Could you check a few things on this model? Use its own coordinates, in mm. Give positions to 0.01 mm unless a question says otherwise; leave off trailing zeros. Order: outer loops, then holes, each group sorted by start corner. A loop starts at its lowest first (then second) coordinate and runs counter-clockwise, first axis right, second up. Notation, with made-up numbers: M 9,11 L 51,11 A21 cw 51,44 Z; hole C 15,80 d11. An arc over 180 degrees is marked long. Answer in a Markdown table with one row per item. Add a question column.
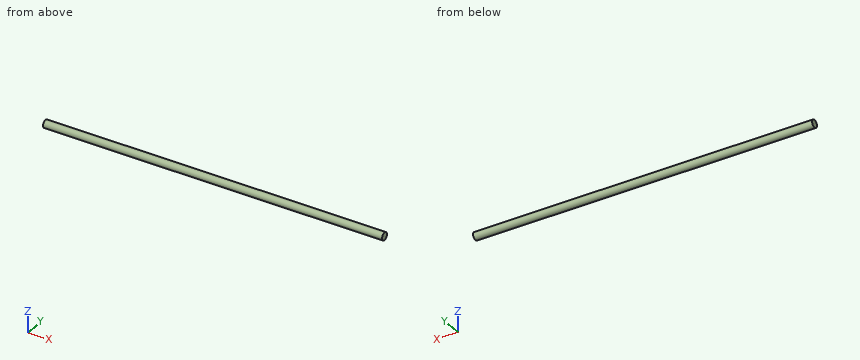
```python
from build123d import *

# Parameters (mm, degrees)
F0_R          = 59.6501704978
F1_DEPTH      = 304.8
F1_DEPTH_BACK = 304.8
F2_R          = 59.6501704978
F2_R_2        = 21.0714216583
F3_DEPTH      = 609.601
F4_R          = 21.0714216583
F4_R_2        = 8.5899800626
F5_DEPTH      = 609.601
F6_DEPTH      = 152.4
F7_DEPTH      = 152.4
F8_DEPTH      = 76.2
F9_DEPTH      = 76.2


with BuildPart() as f1:
    # F0 (on Right) → F1 (new body, two sides)
    with BuildSketch(Plane.YZ) as f1_sk:
        Circle(F0_R)
    extrude(amount=F1_DEPTH)
    extrude(f1_sk.sketch, amount=-F1_DEPTH_BACK)

    # F2 (on face) → F3 (cut, through all)
    with BuildSketch(Plane.YZ.offset(304.8)):
        Circle(F2_R)
        Circle(F2_R_2, mode=Mode.SUBTRACT)
    extrude(amount=-F3_DEPTH, mode=Mode.SUBTRACT)

    # F4 (on face) → F5 (cut, through all)
    with BuildSketch(Plane.YZ.offset(304.8)):
        Circle(F4_R)
        Circle(F4_R_2, mode=Mode.SUBTRACT)
    extrude(amount=-F5_DEPTH, mode=Mode.SUBTRACT)

    # F6 (add): a face of the model
    f6_faces = [f1.faces().sort_by_distance(p)[0] for p in [
        (304.8, 0, 0),
    ]]
    extrude(f6_faces, amount=F6_DEPTH)

    # F7 (add): a face of the model
    f7_faces = [f1.faces().sort_by_distance(p)[0] for p in [
        (-304.8, 0, 0),
    ]]
    extrude(f7_faces, amount=F7_DEPTH)

    # F8 (cut): a face of the model
    f8_faces = [f1.faces().sort_by_distance(p)[0] for p in [
        (457.2, 0, 0),
    ]]
    extrude(f8_faces, amount=-F8_DEPTH, mode=Mode.SUBTRACT)

    # F9 (cut): a face of the model
    f9_faces = [f1.faces().sort_by_distance(p)[0] for p in [
        (-457.2, 0, 0),
    ]]
    extrude(f9_faces, amount=-F9_DEPTH, mode=Mode.SUBTRACT)


solid = f1.part
```
1. Will these pins go through, and if not, where does the flat tip stop? P1, Ø3, axis at x = 229, y = 3, coming from the -Z side; P2, Ø5, axis at x = 81.5, z = 0.5, coming from the +Y side; P3, Ø6, axis at x = 263.5, z = 6.5, coming from the -Y side; P4, Ø1.5, axis at x = -13, y = 6, coming from the +Z side.
2. If I drill on line 1 along Z through (x, y) = (-163.5, -1.25); line 2 along Z through (x, y) = (-262, -0.25); line 3 along Y through (x, z) = (78.5, 0.5), over which ranges is the centre line in solid material (lowest first)? Write a range as [from, to].
3. Suppose I cut it at C-C on z = -2.75. List the corners of the cut face in (x, y) for me, plus the area to 3 significant figures.
4. Suppose I cut it at A-A on x = 37.5. List the corners of the cut face in (y, z) for me, plus the area to 3 significant figures.
5. Suppose I cut it at B-B on y = 1.5. List the corners of the cut face in (x, z) for me, plus the area to 3 significant figures.
Findings below:
| question | item | result |
|---|---|---|
| 1 | P1 | z = -8.46 |
| 1 | P2 | y = 8.59 |
| 1 | P3 | y = -7.84 |
| 1 | P4 | z = 6.8 |
| 2 | line 1 | [-8.5, 8.5] |
| 2 | line 2 | [-8.59, 8.59] |
| 2 | line 3 | [-8.58, 8.58] |
| 3 | outline | M -381,-8.14 L 381,-8.14 L 381,8.14 L -381,8.14 Z |
| 3 | area | 12,400 mm2 |
| 4 | outline | C 0,0 d17.18 |
| 4 | area | 232 mm2 |
| 5 | outline | M -381,-8.46 L 381,-8.46 L 381,8.46 L -381,8.46 Z |
| 5 | area | 12,900 mm2 |
